Work out the finished part from the listing and answer in its coordinate system (mm). A direction names the side the tool comes from. Round coordinates to 2 decimals unless told otherwise and drop trailing zeros. Loops run counter-clockwise (first coordinate to the right, second up) from the corner with the lowest first, then second, coordinate; pieces in that order, holes last. Notation, with made-up numbers: (45, -5) - (63, -5) arc R18 ccw to (63, 30) - close; hole circle Ø6 at (27.25, 58). An arc over 180 degrees is marked (long way). Answer as CSV lines item,"result". Start each with the question number.
Q1. For faces 4 (the face through (51.8, -17.531, 96.155)), 5 (the face through (-85, -18, 107.763)), 6 (the face through (108, 20.32, 1)), determine the directions among +Z, -Z, +X, -X, +Y, -Y from which every point of the face is accessible in a straight line to the end or side of a thin tool.
Q2. Section B-B on y = -14 is taken. Write down the section's boundary in (x, z).
Q3. Section A-A on z = 4 is taken. Write down the section's boundary in (x, y), then the cut area to 3 significant figures.
Q4. Section D-D on x = 90 is taken. Write down the section's boundary in (y, z) (3 decimals), then the cut area to 3 significant figures.
Q5. The mould has two halves that part along Z. Classify faces 1 (the face through (95.825, -17.531, 51.47)), 2 (the face through (2.54, 23, -2)), 3 (the face through (86, -18, 107.763)): +Z half, -Z half, draft (parallel to the pull), parting line (faces both ways), or undercut.
Q6. Each of these flat-tipped pins is pushed along its axis until it touches: pin 1 Ø1.9 at (y, z) = (23, -22) entering from -X; pin 2 Ø6 at (x, y) = (-71, -8.5) entering from -Z; pin 3 Ø16.5 at (x, y) = (120.5, 7) entering from +Z (3 decimals). Where does it stop, or does it pass through?
Q7. Section C-C on x = 145.5 is taken. Write down the section's boundary in (y, z) (3 decimals).
Q8. Straight lines are drawn through the part: L1, parallel to Z at x = -38.1, y = 22.5 (1 decimal); L2, parallel to Y at x = -12, z = -93; L3, parallel to Y at x = 59, z = 75.5. For each, find the intervals that lie inside material, in ascending order. Write a range as [from, to].
```python
from build123d import *

# Parameters (mm, degrees)
F1_DEPTH = 35.56
F2_W     = 254
F2_H     = 158.75
F3_DEPTH = 20.32
F4_W     = 81.28
F4_H     = 250.19
F5_DEPTH = 6.35
F6_D     = 9.525


with BuildPart() as f1:
    # F0 (on Front) → F1 (new body)
    with BuildSketch(Plane.XZ):
        Polygon((107.763073, 63.407903), (107.763073, 107.763073), (63.407903, 107.763073), (39.86235, 84.21752), (0, 84.21752), (-39.86235, 84.21752), (-63.407903, 107.763073), (-107.763073, 107.763073), (-107.763073, 63.407903), (-84.21752, 39.86235), (-84.21752, 0), (-84.21752, -39.86235), (-107.763073, -63.407903), (-107.763073, -107.763073), (-63.407903, -107.763073), (-39.86235, -84.21752), (0, -84.21752), (39.86235, -84.21752), (63.407903, -107.763073), (107.763073, -107.763073), (107.763073, -63.407903), (84.21752, -39.86235), (84.21752, 0), (84.21752, 39.86235), align=None)
    extrude(amount=F1_DEPTH)

    # F2 (on Front) → F3 (join)
    with BuildSketch(Plane.XZ):
        with Locations((88.9, 0)):
            Rectangle(F2_W, F2_H)
    extrude(amount=-F3_DEPTH)

    # F4 (on face) → F5 (join)
    with BuildSketch(Plane(origin=(0, 20.32, 0), x_dir=(-1, 0, 0), z_dir=(0, 1, 0))):
        with Locations((38.1, 0)):
            Rectangle(F4_W, F4_H)
    extrude(amount=F5_DEPTH)

    # F6 (through all)
    with Locations(Plane(origin=(0, 20.32, 0), x_dir=(-1, 0, 0), z_dir=(0, -1, 0))):
        with Locations((38.1, 99.695), (38.1, -99.695)):
            Hole(F6_D / 2)


solid = f1.part
```
Findings:
1,face 4,"+Z, +Y, -Y"
1,face 5,"+Z, +X, -X, -Y"
1,face 6,"+Z, -Z, +X, +Y"
2,outline,"(-107.76, -107.76) - (-63.41, -107.76) - (-39.86, -84.22) - (39.86, -84.22) - (63.41, -107.76) - (107.76, -107.76) - (107.76, -63.41) - (84.22, -39.86) - (84.22, 39.86) - (107.76, 63.41) - (107.76, 107.76) - (63.41, 107.76) - (39.86, 84.22) - (-39.86, 84.22) - (-63.41, 107.76) - (-107.76, 107.76) - (-107.76, 63.41) - (-84.22, 39.86) - (-84.22, -39.86) - (-107.76, -63.41) - close"
3,outline,"(-84.22, -35.56) - (84.22, -35.56) - (84.22, 0) - (215.9, 0) - (215.9, 20.32) - (2.54, 20.32) - (2.54, 26.67) - (-78.74, 26.67) - (-78.74, 20.32) - (-38.1, 20.32) - (-38.1, 0) - (-84.22, 0) - close"
3,area,"11,700 mm^2"
4,outline,"(-35.56, -107.763) - (0, -107.763) - (0, -79.375) - (20.32, -79.375) - (20.32, 79.375) - (0, 79.375) - (0, 107.763) - (-35.56, 107.763) - (-35.56, 45.645) - (0, 45.645) - (0, -45.645) - (-35.56, -45.645) - close"
4,area,"7,640 mm^2"
5,face 1,"undercut"
5,face 2,"draft"
5,face 3,"+Z half"
6,pin 1,"stops at x = -78.74"
6,pin 2,"stops at z = -107.76"
6,pin 3,"stops at z = 79.375"
7,outline,"(0, -79.375) - (20.32, -79.375) - (20.32, 79.375) - (0, 79.375) - close"
8,L1,"z = [-125.1, -104.5], [-94.9, 94.9], [104.5, 125.1]"
8,L2,"y = [20.32, 26.67]"
8,L3,"y = [-35.56, 20.32]"
